```python
from build123d import *

# Parameters (mm, degrees)
SKETCH_8_W      = 80
SKETCH_8_H      = 60
SKETCH_8_W_2    = 68
SKETCH_8_H_2    = 48
EXTRUDE_1_DEPTH = 175
SKETCH_9_W      = 100
SKETCH_9_H      = 80
SKETCH_9_R      = 20
EXTRUDE_2_DEPTH = 12
EXTRUDE_START   = 12
SKETCH_10_W     = 100
SKETCH_10_H     = 80
SKETCH_10_R     = 20
EXTRUDE_3_DEPTH = 12


with BuildPart() as part:
    # 草图8 → 凸台-拉伸1 (new, symmetric)
    with BuildSketch(Plane.XY):
        Rectangle(SKETCH_8_W, SKETCH_8_H)
        Rectangle(SKETCH_8_W_2, SKETCH_8_H_2, mode=Mode.SUBTRACT)
    extrude(amount=EXTRUDE_1_DEPTH, both=True)

    # 草图9 → 凸台-拉伸2 (add)
    with BuildSketch(Plane.XY.offset(175)):
        Rectangle(SKETCH_9_W, SKETCH_9_H)
        Circle(SKETCH_9_R, mode=Mode.SUBTRACT)
    extrude(amount=EXTRUDE_2_DEPTH)

    # 草图10 → 凸台-拉伸3 (add)
    with BuildSketch(Plane(origin=(0, 0, -175), x_dir=(-1, 0, 0), z_dir=(0, 0, -1)).offset(EXTRUDE_START)):
        Rectangle(SKETCH_10_W, SKETCH_10_H)
        with Locations(Location((0, 0, 0), (0, 0, 180))):
            Circle(SKETCH_10_R, mode=Mode.SUBTRACT)
    extrude(amount=-EXTRUDE_3_DEPTH)


solid = part.part
```
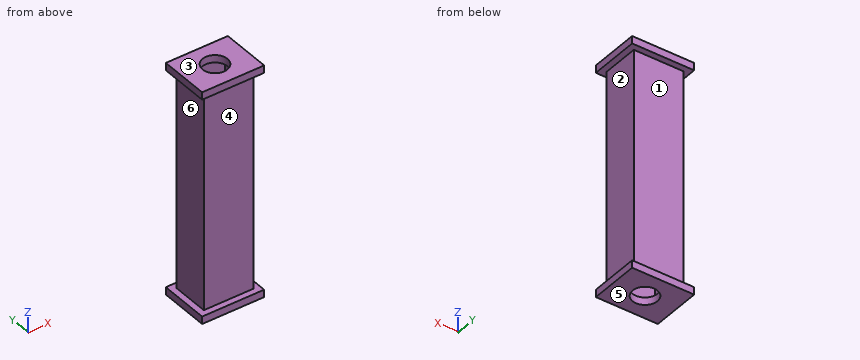
Input: part model. Units: mm. Frame: model coordinates. Face numbers are marked on the shaded views. A direction names the side the tool comes from. Give positions to 0.01 mm unless a question says otherwise; leave off trailing zeros. Order: outer loops, then holes, each group sorted by start corner. A loop starts at its lowest first (then second) coordinate and runs counter-clockwise, first axis right, second up. Notation, with made-up numbers: (18.5, -32.75) - (65.5, -32.75) arc R33 cw to (65.5, 2.25) - close; hole circle Ø3 at (53, 37.25). An arc over 180 degrees is marked (long way). Put each result on its own line as item: value.
Item 1: Draft query along Z for the marked faces 3, 4, 5 and 6. Return one class per face: +Z half, -Z half, draft (parallel to the pull), parting line (faces both ways), or undercut.
Found:
face 3: +Z half
face 4: undercut
face 5: -Z half
face 6: undercut
Item 2: Section query B-B, the plane x = 0. Return loops of the section in (y, z), then the cut area to 3 significant figures.
Found:
outline: (-40, -187) - (-20, -187) - (-20, -175) - (-24, -175) - (-24, 175) - (-20, 175) - (-20, 187) - (-40, 187) - (-40, 175) - (-30, 175) - (-30, -175) - (-40, -175) - close; (20, -187) - (40, -187) - (40, -175) - (30, -175) - (30, 175) - (40, 175) - (40, 187) - (20, 187) - (20, 175) - (24, 175) - (24, -175) - (20, -175) - close
area: 5,160 mm^2
Item 3: Section query A-A, the plane y = -34.5. Return loops of the section in (x, z).
Found:
outline: (-50, -187) - (50, -187) - (50, -175) - (-50, -175) - close; (-50, 175) - (50, 175) - (50, 187) - (-50, 187) - close
Item 4: Section query C-C, the plane z = -114.5. Return loops of the section in (x, y), then the cut area to 3 significant figures.
Found:
outline: (-40, -30) - (40, -30) - (40, 30) - (-40, 30) - close; hole (-34, -24) - (34, -24) - (34, 24) - (-34, 24) - close
area: 1,540 mm^2
Item 5: Contact query for flat-ended pins moving along their axis: pin 1 (24 mm diameter, centred on y = 1.5, z = -60, fed in from +X); pin 2 (4 mm diameter, centred on x = 31.5, z = 88, fed in from -Y); pin 3 (20.5 mm diameter, centred on x = -9.5, z = -1, fed in from +Y). Output: stop coordinate, or through.
Found:
pin 1: stops at x = 40
pin 2: stops at y = -30
pin 3: stops at y = 30
Item 6: Access query for the marked faces 1 and 2. Directions: +Z, -Z, +X, -X, +Y, -Y. A direction counts if a zero-diameter tool reaches every point of the face in a straight line with its end or side. Return the directions, or none.
Found:
face 1: +X, -X, +Y
face 2: +X, +Y, -Y
Item 7: Ray query, L1, parallel to Y at x = -3.5, z = -105; L2, parallel to Z at x = 40, y = -33; L3, parallel to X at y = -16, z = 157.5. Return the intervals inside material, ascending. Write a range as from..to.
Found:
L1: y = -30..-24, 24..30
L2: z = -187..-175, 175..187
L3: x = -40..-34, 34..40
Item 8: Section query D-D, the plane y = 0. Return loops of the section in (x, z), then the cut area to 3 significant figures.
Found:
outline: (-50, -187) - (-20, -187) - (-20, -175) - (-34, -175) - (-34, 175) - (-20, 175) - (-20, 187) - (-50, 187) - (-50, 175) - (-40, 175) - (-40, -175) - (-50, -175) - close; (20, -187) - (50, -187) - (50, -175) - (40, -175) - (40, 175) - (50, 175) - (50, 187) - (20, 187) - (20, 175) - (34, 175) - (34, -175) - (20, -175) - close
area: 5,640 mm^2
